Source: CAD feature listing. Evaluate the final solid. Frame: model axes, mm. A direction names the side the tool comes from. Round coordinates to 2 decimals unless told otherwise and drop trailing zeros. Write each loop counter-clockwise with the first axis right and the second up, starting at its lowest first coordinate (ties: lowest second). Pieces come first, ordered by that corner, then holes. Notation, with made-up numbers: M 40.25,30.25 L 62.25,30.25 A21 cw 62.25,35.25 Z; hole C 80.5,86.5 d1. An arc over 180 degrees is marked long. Answer in a Markdown table with one row per item.
from build123d import *

# Parameters (mm, degrees)
SKETCH1_W           = 28
SKETCH1_H           = 17.5
BOSS_EXTRUDE1_DEPTH = 10
SKETCH3_W           = 4.6
SKETCH3_H           = 12
CUT_EXTRUDE1_DEPTH  = 8.6
SKETCH4_R           = 3.05
BOSS_EXTRUDE2_DEPTH = 4.2
SKETCH5_R           = 2
BOSS_EXTRUDE3_DEPTH = 5
FILLET1_R           = 1.5


with BuildPart() as part:
    # Sketch1 → Boss-Extrude1 (new body)
    with BuildSketch(Plane.XY):
        with Locations((14, 8.75)):
            Rectangle(SKETCH1_W, SKETCH1_H)
    extrude(amount=BOSS_EXTRUDE1_DEPTH)

    # Sketch3 → Cut-Extrude1 (cut)
    with BuildSketch(Plane.ZY):
        with Locations((5, 8.75)):
            Rectangle(SKETCH3_W, SKETCH3_H)
    extrude(amount=-CUT_EXTRUDE1_DEPTH, mode=Mode.SUBTRACT)

    # Sketch4 → Boss-Extrude2 (add)
    with BuildSketch(Plane(origin=(28, 0, 0), x_dir=(0, 0, -1), z_dir=(1, 0, 0))):
        with Locations((-5, 8.75)):
            Circle(SKETCH4_R)
    extrude(amount=BOSS_EXTRUDE2_DEPTH)

    # Sketch5 → Boss-Extrude3 (add)
    with BuildSketch(Plane(origin=(32.2, 0, 0), x_dir=(0, 0, -1), z_dir=(1, 0, 0))):
        with Locations((-5, 8.75)):
            Circle(SKETCH5_R)
    extrude(amount=BOSS_EXTRUDE3_DEPTH)

    # Fillet1
    fillet1_edges = [part.edges().sort_by_distance(p)[0] for p in [
        (14, 17.5, 10),
        (14, 17.5, 0),
        (14, 0, 0),
        (14, 0, 10),
    ]]
    fillet(fillet1_edges, radius=FILLET1_R)


solid = part.part
Q1. Pull-direction query (Y, two-part tool) for faces 1 (the flat face through (8.6, 9, 5)), 2 (the cylindrical face through (14.2, 17.05, 0.43)), 3 (the flat face through (28, 8.6, 1.6)), 4 (the flat face through (4, 9, 7.3)); classes: pulls with the +Y half, pulls with the -Y half, needs draft (parallel to the pull), parting line crosses it, or undercut.
Solutions:
| item | result |
|---|---|
| face 1 | undercut |
| face 2 | pulls with the +Y half |
| face 3 | needs draft |
| face 4 | undercut |
Q2. Section D-D (x = 29). Return loops of the section in (y, z).
Solutions:
| item | result |
|---|---|
| outline | C 8.75,5 d6.1 |
Q3. Contact query for flat-ended pins moving along their axis: pin 1 Ø5 at (y, z) = (12.5, 5) entering from +X; pin 2 Ø1 at (x, y) = (33, 8) entering from +Z. Output: stop coordinate, or through.
Solutions:
| item | result |
|---|---|
| pin 1 | stops at x = 37.2 |
| pin 2 | stops at z = 6.98 |
Q4. Section C-C (z = 5). Return loops of the section in (x, y), and give its area (3 significant figures).
Solutions:
| item | result |
|---|---|
| outline | M 0,0 L 28,0 L 28,5.7 L 32.2,5.7 L 32.2,6.75 L 37.2,6.75 L 37.2,10.75 L 32.2,10.75 L 32.2,11.8 L 28,11.8 L 28,17.5 L 0,17.5 L 0,14.75 L 8.6,14.75 L 8.6,2.75 L 0,2.75 Z |
| area | 432 mm2 |
Q5. Section A-A (x = 4.5). Return loops of the section in (y, z), and give its area (3 significant figures).
Solutions:
| item | result |
|---|---|
| outline | M 0,1.5 A1.5 ccw 1.5,0 L 16,0 A1.5 ccw 17.5,1.5 L 17.5,8.5 A1.5 ccw 16,10 L 1.5,10 A1.5 ccw 0,8.5 Z; hole M 2.75,2.7 L 14.75,2.7 L 14.75,7.3 L 2.75,7.3 Z |
| area | 118 mm2 |
Q6. Section B-B (y = 8.75). Return loops of the section in (x, z), and give its area (3 significant figures).
Solutions:
| item | result |
|---|---|
| outline | M 0,0 L 28,0 L 28,1.95 L 32.2,1.95 L 32.2,3 L 37.2,3 L 37.2,7 L 32.2,7 L 32.2,8.05 L 28,8.05 L 28,10 L 0,10 L 0,7.3 L 8.6,7.3 L 8.6,2.7 L 0,2.7 Z |
| area | 286 mm2 |
Q7. Material intervals for probe 1 along Z at (x, y) = (4, 3.25); probe 2 along X at (y, z) = (13, 2.25); probe 3 along X at (y, z) = (5, 6.5), sorted ascending.
Solutions:
| item | result |
|---|---|
| probe 1 | z = 0 to 2.7, 7.3 to 10 |
| probe 2 | x = 0 to 28 |
| probe 3 | x = 8.6 to 28 |
Q8. Access query for faces 5 (the cylindrical face through (34.665, 10.733, 5.26)), 6 (the flat face through (0, 9, 2)), 7 (the flat face through (4, 2.75, 5)). Directions: +Z, -Z, +X, -X, +Y, -Y. A direction counts if a zero-diameter tool reaches every point of the face in a straight line with its end or side. Return the directions, or none.
Solutions:
| item | result |
|---|---|
| face 5 | +X |
| face 6 | +Z, -Z, -X, +Y, -Y |
| face 7 | -X |
